Read the model definition and answer for the solid it produces. Units are mm, in the model's axes. A direction names the side the tool comes from. Round coordinates to 2 decimals unless told otherwise and drop trailing zeros. Write each loop counter-clockwise with the first axis right and the second up, starting at its lowest first coordinate (ties: lowest second). Pieces come first, ordered by that corner, then holes. Notation, with made-up numbers: (-26.5, -13.5) -> (-19.5, -13.5) arc R11 ccw to (-19.5, -6.5) -> close; hole circle Ø4 at (-9.5, 84.5). An arc over 180 degrees is marked (long way). Return JSON: item names as keys, results as strings. Group by question number.
(1) A cutting plane is placed at C-C on z = -8.5. Give the vertices of the cut face in (x, y).
(2) A cutting plane is placed at A-A on x = 5. Give the vertices of the cut face in (y, z).
(3) Given pin 1 (2.5 mm diameter, centred on x = -16.51, y = 20.42, fed in from -Z); pin 2 (3.5 mm diameter, centred on x = 15, y = 20.5, fed in from -Z); pin 3 (1 mm diameter, centred on x = -5, z = -6, fed in from -Y), each flat-ended and moving along its own axis, determine where each tip first touches the part or whether it passes through.
(4) The mould has two halves that part along Y. Classify faces 1 (the flat face through (-1, 25.922, 15)), 2 (the cylindrical face through (15.598, 21.436, 2.465)), 3 (the flat face through (-1, 5, -22)): released by +Y, released by -Y, zero draft, split by the parting line, or undercut.
(5) For faces 4 (the flat face through (-22.008, 5, 15)), 5 (the flat face through (-11, 15, 0)), determine the directions among +Z, -Z, +X, -X, +Y, -Y from which every point of the face is accessible in a straight line to the end or side of a thin tool.
(6) A cutting plane is placed at D-D on y = -8. Give the vertices of the cut face in (x, z).
(7) Straight lines are drawn through the part: line 1 (Z direction, x = 4.5, y = 2); line 2 (Z direction, x = -14, y = 3.5); line 3 (Y direction, x = -2.5, z = -0.5). For each, find the intervals that lie inside material, in ascending order.
(8) A cutting plane is placed at B-B on y = 9. Give the vertices of the cut face in (x, z), then the cut area to 3 significant figures.
Autodesk Inventor part; units mm, degrees
ref_plane "YZ Plane" through (0, 0, 0) normal (1, 0, 0) x (0, 1, 0)
ref_plane "XZ Plane" through (0, 0, 0) normal (0, 1, 0) x (-1, 0, 0)
ref_plane "XY Plane" through (0, 0, 0) normal (0, 0, 1) x (1, 0, 0)
sketch "Sketch1" plane through (0, 0, 0) normal (0, 0, 1) x (1, 0, 0)
  line L0 (19.9924, -21.8579) -> (16.7724, -25.0779)
  line L1 (19.9924, -21.8579) -> (19.9924, 20.4221)
  arc A0 (19.9924, 20.4221) -> (14.4924, 25.9221) centre (14.4924, 20.4221) ccw construction
  line L2 (14.4924, 25.9221) -> (14.2174, 25.9221)
  line L3 (14.2174, 25.9221) -> (14.2174, 26.4221)
  line L4 (9.7174, 30.9221) -> (14.2174, 26.4221)
  line L5 (-3.2826, 30.9221) -> (3.2174, 30.9221)
  line L6 (-7.7826, 26.4221) -> (-3.2826, 30.9221)
  line L7 (-7.7826, 25.9221) -> (-7.7826, 26.4221)
  line L8 (-7.7826, 25.9221) -> (-16.5076, 25.9221)
  arc A1 (-16.5076, 25.9221) -> (-22.0076, 20.4221) centre (-16.5076, 20.4221) ccw construction
  line L9 (-22.0076, 20.4221) -> (-22.0076, -10.5779)
  arc A2 (-22.0076, -10.5779) -> (-16.5076, -16.0779) centre (-16.5076, -10.5779) ccw construction
  line L10 (-16.5076, -16.0779) -> (-13.0076, -16.0779)
  line L11 (-13.0076, -16.0779) -> (-13.0076, -21.8579)
  line L12 (-9.7876, -25.0779) -> (-13.0076, -21.8579)
  line L13 (-9.7876, -25.0779) -> (-9.7826, -25.0779)
  line L14 (-12.7826, -28.0779) -> (-9.7826, -25.0779)
  line L15 (-15.5326, -28.0779) -> (-12.7826, -28.0779)
  line L16 (-15.5326, -28.0779) -> (-15.5326, -66.0779)
  arc A3 (-15.5326, -66.0779) -> (-9.5326, -72.0779) centre (-9.5326, -66.0779) ccw
  line L17 (-9.5326, -72.0779) -> (15.9674, -72.0779)
  arc A4 (15.9674, -72.0779) -> (21.9674, -66.0779) centre (15.9674, -66.0779) ccw
  line L18 (21.9674, -28.0779) -> (21.9674, -66.0779)
  line L19 (19.2174, -28.0779) -> (21.9674, -28.0779)
  line L20 (19.2174, -28.0779) -> (16.2174, -25.0779)
  line L21 (16.2174, -25.0779) -> (16.7724, -25.0779)
  circle A5 centre (-16.5076, 20.4221) radius 1.7 construction
  circle A6 centre (14.4924, 20.4221) radius 1.7 construction
  circle A7 centre (14.4924, -10.5779) radius 1.7 construction
  circle A8 centre (-16.5076, -10.5779) radius 1.7 construction
  circle A9 centre (14.7174, -41.5779) radius 2.25
  circle A10 centre (-8.2826, -41.5779) radius 2.25
  circle A11 centre (14.7174, -64.5779) radius 2.25
  circle A12 centre (-8.2826, -64.5779) radius 2.25
  circle A13 centre (-1.0076, 4.9221) radius 12.5 construction
  line L22 (-20.0076, 25.9221) -> (17.9924, 25.9221)
  line L23 (19.9924, 23.9221) -> (19.9924, -14.0779)
  line L24 (17.9924, -16.0779) -> (-20.0076, -16.0779)
  line L25 (-22.0076, -14.0779) -> (-22.0076, 23.9221)
  line L26 (-22.0076, 25.9221) -> (19.9924, -16.0779) construction
  line L27 (19.9924, 25.9221) -> (-22.0076, -16.0779) construction
  line L28 (-20.0076, 25.9221) -> (-22.0076, 23.9221)
  line L29 (17.9924, 25.9221) -> (19.9924, 23.9221)
  line L30 (19.9924, -14.0779) -> (17.9924, -16.0779)
  line L31 (-20.0076, -16.0779) -> (-22.0076, -14.0779)
  line L32 (7.7174, 40.9221) -> (8.8956, 39.0987)
  line L33 (5.2174, 40.9221) -> (7.7174, 40.9221)
  line L34 (3.2174, 38.9221) -> (5.2174, 40.9221)
  line L35 (3.2174, 30.9221) -> (3.2174, 38.9221)
  arc A14 (8.8956, 39.0987) -> (9.7174, 30.9221) centre (18.3776, 35.9221) ccw
  point P0 (0, 0)
  dimension "d0" = 2
  dimension "d1" = 2
  dimension "d2" = 2
  dimension "d3" = 2
  dimension "d4" = 2
  dimension "d5" = 2
  dimension "d6" = 2
  dimension "d7" = 2
extrude "Extrusion1" add sketch "Sketch1" along normal blind 31 contours L30 L24 L10 L31 L25 L9 L28 L22 L8 L2 L29 L23 L1
sketch "Sketch2" plane through (0, 0, 0) normal (0, 0, -1) x (-1, 0, 0)
  circle A0 centre (1.0076, 4.9221) radius 12.5
  circle A1 centre (1.0076, 4.9221) radius 11
  point P0 (0, 0)
  dimension "d10" = 22
extrude "Extrusion2" add sketch "Sketch2" along normal blind 2 contours A1
sketch "Sketch3" plane through (0, 0, 0) normal (0, 0, -1) x (-1, 0, 0)
  line L0 (20.0076, 25.9221) -> (22.0076, 23.9221)
  line L1 (-19.9924, 23.9221) -> (-17.9924, 25.9221)
  line L2 (-17.9924, -16.0779) -> (-19.9924, -14.0779)
  line L3 (22.0076, -14.0779) -> (20.0076, -16.0779)
  circle A0 centre (-14.4924, 20.4221) radius 1.5
  circle A1 centre (16.5076, 20.4221) radius 1.5
  line L4 (-18.9924, 24.9221) -> (21.0076, -15.0779) construction
  line L5 (21.0076, 24.9221) -> (-18.9924, -15.0779) construction
  circle A2 centre (-14.4924, -10.5779) radius 1.5
  circle A3 centre (16.5076, -10.5779) radius 1.5
  point P0 (0, 0)
  dimension "d13" = 31
  dimension "d14" = 3
extrude "Extrusion3" cut sketch "Sketch3" against normal blind 5
sketch "Sketch4" plane through (-1.0076, 4.9221, -2) normal (0, 0, -1) x (-1, 0, 0)
  circle A0 centre (0, 0) radius 11
  circle A1 centre (0, 0) radius 2.5
  point P0 (-1.0076, -4.9221)
  dimension "d17" = 5
extrude "Extrusion4" add sketch "Sketch4" along normal blind 20 contours A1
equation "\"d1\" = d0"
equation "\"d2\" = d0"
equation "\"d3\" = d2"
equation "\"d4\" = d0"
equation "\"d5\" = d4"
equation "\"d6\" = d0"
equation "\"d7\" = d6"
properties part number "NEMA17"
Checks:
{
 "1": {"outline": "circle Ø5 at (-1.01, 4.92)"},
 "2": {"outline": "(-16.08, 0) -> (-4.29, 0) -> (-4.29, -2) -> (14.14, -2) -> (14.14, 0) -> (25.92, 0) -> (25.92, 31) -> (-16.08, 31) -> close"},
 "3": {"pin 1": "stops at z = 5", "pin 2": "stops at z = 0", "pin 3": "passes through"},
 "4": {"face 1": "released by +Y", "face 2": "undercut", "face 3": "zero draft"},
 "5": {"face 4": "+Z, -Z, -X, +Y, -Y", "face 5": "-Z"},
 "6": {"outline": "(-22.01, 0) -> (19.99, 0) -> (19.99, 31) -> (-22.01, 31) -> close"},
 "7": {"line 1": "z = -2 to 31", "line 2": "z = 0 to 31", "line 3": "y = -5.98 to 15.82"},
 "8": {"outline": "(-22.01, 0) -> (-11.22, 0) -> (-11.22, -2) -> (9.21, -2) -> (9.21, 0) -> (19.99, 0) -> (19.99, 31) -> (-22.01, 31) -> close", "area": "1,340 mm^2"}
}
